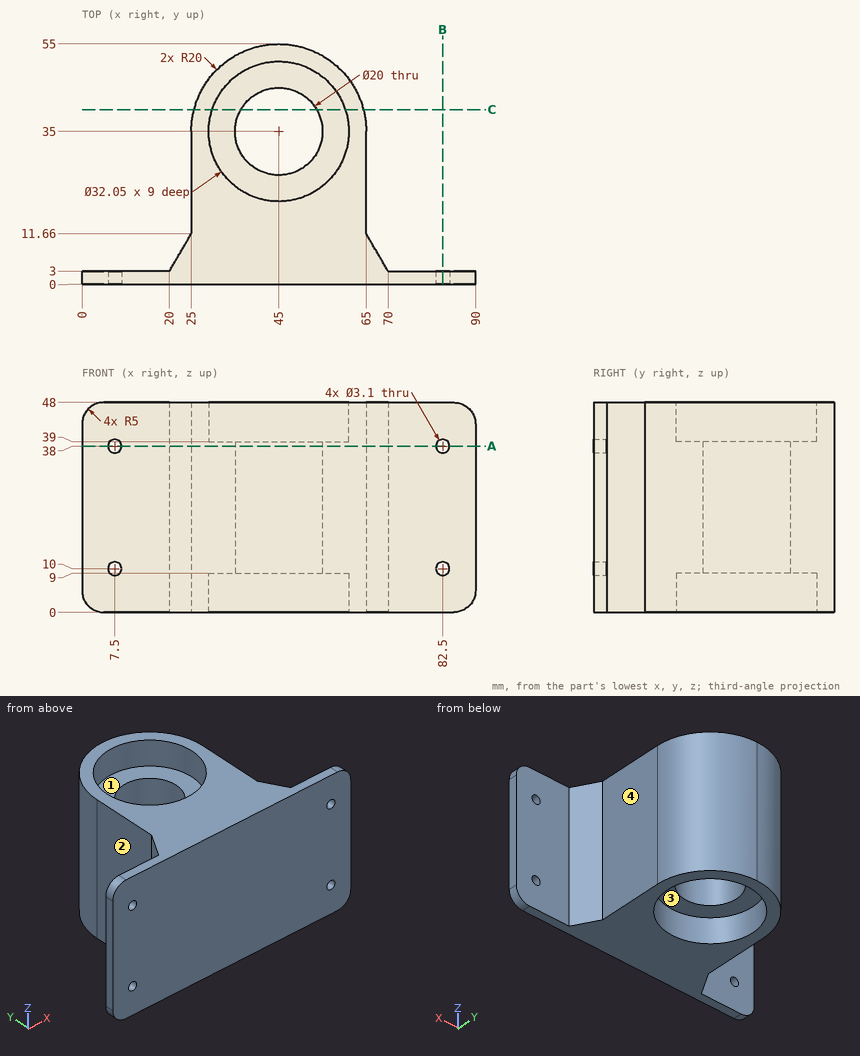
Check sheet for the drawn part. Datum: minimum x, y, z corner. Units: mm. A direction names the side the tool comes from. Round coordinates to 2 decimals unless told otherwise and drop trailing zeros. Write each loop counter-clockwise with the first axis right and the second up, starting at its lowest first coordinate (ties: lowest second). Pieces come first, ordered by that corner, then holes. Notation, with made-up numbers: (32, 69.25) -> (91, 69.25) arc R21 cw to (91, 82.25) -> close; hole circle Ø4 at (62.5, 69). An arc over 180 degrees is marked (long way). Write each question's results on one line, items separated by ' | '. Start each with the question number.
1. Set-up check for the marked faces 1, 2, 3 and 4: record each of +Z, -Z, +X, -X, +Y, -Y from which the full face is reachable in a straight line by a thin tool's end or side.
2. Material ranges on probe 1 along X at (y, z) = (1.5, 38); probe 2 along Z at (x, y) = (7.5, 1.9); probe 3 along Y at (x, z) = (45, 25.25), recorded low to high. Write a range as from..to.
3. Cross-section at C-C (y = 40). Enter the section's corners in (x, z) (1 decimal), then the cut area to 3 significant figures.
4. Cross-section at A-A (z = 38). Count the separate pieces of the cut face and the enclosed holes in it, then the cut area to 3 significant figures.
5. Cross-section at B-B (x = 82.5). Enter the section's corners in (y, z), then the cut area to 3 significant figures.
6. Depth check by flat-ended pin: P1, Ø16, axis at x = 79, z = 32.5, coming from the +Y side; P2, Ø9.5, axis at x = 51, y = 27, coming from the +Z side; P3, Ø11.5, axis at y = 27.5, z = 17.5, coming from the +X side. Enter the tip coordinate at first touch or a pass-through.
Solutions:
1) face 1: +Z | face 2: +Z, -Z, -X, +Y | face 3: -Z | face 4: +Z, -Z, +X, +Y
2) probe 1: x = 0..5.95, 9.05..80.95, 84.05..90 | probe 2: z = 0..8.45, 11.55..36.45, 39.55..48 | probe 3: y = 0..25, 45..55
3) outline: (25.6, 0) -> (29.8, 0) -> (29.8, 9) -> (36.3, 9) -> (36.3, 39) -> (29.8, 39) -> (29.8, 48) -> (25.6, 48) -> close; (53.7, 9) -> (60.2, 9) -> (60.2, 0) -> (64.4, 0) -> (64.4, 48) -> (60.2, 48) -> (60.2, 39) -> (53.7, 39) -> close | area: 791 mm2
4) separate pieces: 3 | enclosed holes: 1 | area: 1,890 mm2
5) outline: (0, 0) -> (3, 0) -> (3, 8.45) -> (0, 8.45) -> close; (0, 11.55) -> (3, 11.55) -> (3, 36.45) -> (0, 36.45) -> close; (0, 39.55) -> (3, 39.55) -> (3, 48) -> (0, 48) -> close | area: 125 mm2
6) P1: stops at y = 3 | P2: stops at z = 39 | P3: stops at x = 65
